Autodesk Inventor part; units mm, degrees
ref_plane "YZ Plane" through (0, 0, 0) normal (1, 0, 0) x (0, 1, 0)
ref_plane "XZ Plane" through (0, 0, 0) normal (0, 1, 0) x (-1, 0, 0)
ref_plane "XY Plane" through (0, 0, 0) normal (0, 0, 1) x (1, 0, 0)
sketch "Sketch1" plane through (0, 0, 0) normal (0, 0, 1) x (1, 0, 0)
  line L0 (-20.7162, 13.5128) -> (19.2838, 13.5128)
  line L1 (19.2838, 13.5128) -> (19.2838, -66.4872)
  line L2 (19.2838, -66.4872) -> (-20.7162, -66.4872)
  line L3 (-20.7162, -66.4872) -> (-20.7162, 13.5128)
  point P0 (0, 0)
  dimension "d0" = 40
  dimension "d1" = 80
extrude "Extrusion1" add sketch "Sketch1" along normal blind 40
fillet "Fillet1" radius 15 4 edges at (-20.7162, 13.5128, 20) (19.2838, 13.5128, 20) (-20.7162, -66.4872, 20) (19.2838, -66.4872, 20)
shell "Shell1" thickness 2 removed faces 0
ref_plane "Work Plane1" through (0, 0, 34) normal (0, 0, 1) x (1, 0, 0)
sketch "Sketch3" plane through (0, 0, 34) normal (0, 0, 1) x (1, 0, 0)
  arc A0 (-5.7162, 13.5128) -> (-20.7162, -1.4872) centre (-5.7162, -1.4872) ccw
  line L0 (-20.7162, -1.4872) -> (-20.7162, -51.4872)
  line L1 (-20.7162, -51.4872) -> (0, -51.4872)
  line L2 (0, -51.4872) -> (0, 13.5128)
  line L3 (0, 13.5128) -> (-5.7162, 13.5128)
  point P0 (0, 0)
extrude "Extrusion2" cut sketch "Sketch3" against normal blind 15
fillet "Fillet3" radius 2 4 edges at (0, 12.5128, 19) (0, 12.5128, 34) (-19.7162, -51.4872, 34) (-19.7162, -51.4872, 19)
sketch "Sketch4" plane through (0, 0, 40) normal (0, 0, 1) x (1, 0, 0)
  circle A0 centre (-0.7162, -46.4872) radius 2.1395
  circle A1 centre (-0.7162, -6.4872) radius 2.337
  line L0 (-20.7162, -1.4872) -> (-20.7162, -51.4872)
  line L1 (4.2838, 13.5128) -> (-5.7162, 13.5128)
  line L2 (-5.7162, -66.4872) -> (4.2838, -66.4872)
  point P0 (0, 0)
  dimension "d11" = 20
  dimension "d12" = 20
  dimension "d13" = 20
  dimension "d14" = 20
extrude "Extrusion3" cut sketch "Sketch4" against normal up to next
fillet "Fillet4" radius 1 8 edges at (-0.7162, 13.5128, 0) (-16.3228, 9.1194, 0) (-20.7162, -26.4872, 0) (-16.3228, -62.0938, 0) (-0.7162, -66.4872, 0) (14.8904, -62.0938, 0) (19.2838, -26.4872, 0) (14.8904, 9.1194, 0)
properties part number "lock-case"
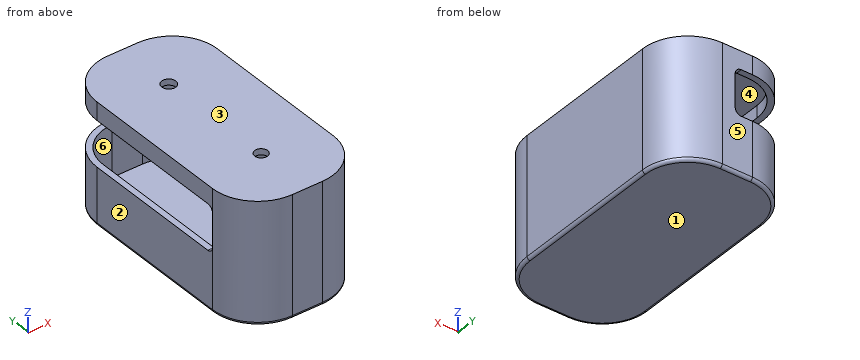
Geometry: final body of the model. Coordinates: model frame, mm. Face numbers are marked on the shaded views. A direction names the side the tool comes from. Coordinates: 2 decimals unless noted, no trailing zeros. Order: outer loops, then holes, each group sorted by start corner. A loop starts at its lowest first (then second) coordinate and runs counter-clockwise, first axis right, second up. Notation, with made-up numbers: (-12.5, 21) - (35.5, 21) arc R25 ccw to (35.5, 60) - close; hole circle Ø1 at (36.25, -0.75). An arc over 180 degrees is marked (long way). Use one line per item in the form item = value.
1) Mould query, pull axis Z, two halves, no side actions, for the marked faces 1, 2, 3 and 4. Classes: +Z half, -Z half, draft (parallel to the pull), parting line (faces both ways), or undercut.
Solutions:
face_1 = -Z half
face_2 = draft
face_3 = +Z half
face_4 = undercut
2) Pin query (flat end, axial travel): pin 1 (2 mm diameter, centred on y = -7, z = 33.5, fed in from -X); pin 2 (2 mm diameter, centred on x = 9.5, z = 26.5, fed in from -Y); pin 3 (1 mm diameter, centred on x = -20, z = 29, fed in from +Y); pin 4 (1 mm diameter, centred on x = -11, z = 36, fed in from +Y). Return the tip coordinate at first contact, or that it passes through.
Solutions:
pin_1 = -20.72
pin_2 = -65.88
pin_3 = -51.49
pin_4 = 12.73
3) Section C-C (z = 24). Return loops of the section in (x, y), then the cut area to 3 significant figures.
Solutions:
outline = (-20.72, -51.49) arc R15 ccw to (-5.72, -66.49) - (4.28, -66.49) arc R15 ccw to (19.28, -51.49) - (19.28, -1.49) arc R15 ccw to (4.28, 13.51) - (0, 13.51) - (0, 11.51) - (4.28, 11.51) arc R13 cw to (17.28, -1.49) - (17.28, -51.49) arc R13 cw to (4.28, -64.49) - (-5.72, -64.49) arc R13 cw to (-18.72, -51.49) - close
area = 261 mm^2
4) Ray query, L1, parallel to Z at x = -1, y = -17; L2, parallel to X at y = -35.5, z = 16.5; L3, parallel to Y at x = 3, z = 8.5. Return the intervals inside material, ascending.
Solutions:
L1 = 0 to 2, 38 to 40
L2 = -20.72 to -18.72, 17.28 to 19.28
L3 = -66.49 to -64.49, 11.51 to 13.51
5) Set-up query: the marked faces 5 and 6. Return all of +Z, -Z, +X, -X, +Y, -Y with unobstructed straight access to the full face (end or side cutting, diameter ignored); none if empty.
Solutions:
face_5 = +Z, -Z, +X, -X, +Y
face_6 = none
6) Section A-A (z = 16.5). Return loops of the section in (x, y), then the cut area to 3 significant figures.
Solutions:
outline = (-20.72, -51.49) arc R15 ccw to (-5.72, -66.49) - (4.28, -66.49) arc R15 ccw to (19.28, -51.49) - (19.28, -1.49) arc R15 ccw to (4.28, 13.51) - (-5.72, 13.51) arc R15 ccw to (-20.72, -1.49) - close; hole (-18.72, -51.49) arc R13 ccw to (-5.72, -64.49) - (4.28, -64.49) arc R13 ccw to (17.28, -51.49) - (17.28, -1.49) arc R13 ccw to (4.28, 11.51) - (-5.72, 11.51) arc R13 ccw to (-18.72, -1.49) - close
area = 416 mm^2
7) Section B-B (y = -32.5). Return loops of the section in (x, z).
Solutions:
outline = (-20.72, 1) arc R1 ccw to (-19.72, 0) - (18.28, 0) arc R1 ccw to (19.28, 1) - (19.28, 40) - (-20.72, 40) - (-20.72, 34) - (-18.72, 34) - (-18.72, 38) - (17.28, 38) - (17.28, 2) - (-18.72, 2) - (-18.72, 19) - (-20.72, 19) - close
